Work out the finished part from the listing and answer in its coordinate system (mm). Face numbers are marked on the shaded views. A direction names the side the tool comes from. Give positions to 0.01 mm unless a question says otherwise; leave off trailing zeros. Order: outer loops, then holes, each group sorted by start corner. A loop starts at its lowest first (then second) coordinate and runs counter-clockwise, first axis right, second up. Notation, with made-up numbers: M 25.5,72.25 L 38.5,72.25 A29 cw 38.5,95.25 Z; hole C 72,48.5 d1. An arc over 180 degrees is marked long. One line per item, written item: value.
Autodesk Fusion 360 part; units mm, degrees
sketch "Sketch1" plane through (0, 0, 0) normal (0, 0, 1) x (1, 0, 0)
  line L0 (0, 0) -> (101.6, 0)
  line L1 (101.6, 0) -> (101.6, -76.2)
  line L2 (101.6, -76.2) -> (0, -76.2)
  line L3 (0, -76.2) -> (0, 0)
  line L4 (101.6, 0) -> (126.0466, 6.8938)
  line L5 (126.0466, 6.8938) -> (176.8466, 6.8938)
  line L6 (176.8466, 6.8938) -> (201.2932, 0)
  line L7 (201.2932, 0) -> (201.2932, -76.2)
  line L8 (201.2932, -76.2) -> (176.8466, -82.9718)
  line L9 (176.8466, -82.9718) -> (126.0466, -82.9718)
  line L10 (126.0466, -82.9718) -> (101.6, -76.2)
  dimension "d1" = 101.6
  dimension "d2" = 76.2
  dimension "d3" = 25.4
  dimension "d4" = 50.8
  dimension "d5" = 25.4
extrude "Extrude1" add sketch "Sketch1" along normal blind 12.7
fillet "Fillet1" radius 11.43 2 edges at (201.2932, -76.2, 6.35) (201.2932, 0, 6.35)
sketch "Sketch2" plane through (0, 0, 12.7) normal (0, 0, 1) x (-1, 0, 0)
  arc A0 (-201.2932, 8.6526) -> (-192.9654, -2.3484) centre (-189.8632, 8.6526) ccw
  line L0 (-192.9654, -2.3484) -> (-176.8466, -6.8938)
  line L1 (-176.8466, -6.8938) -> (-126.0466, -6.8938)
  line L2 (-126.0466, -6.8938) -> (-101.6, 0)
  line L3 (-101.6, 0) -> (0, 0)
  line L4 (0, 0) -> (0, 76.2)
  line L5 (0, 76.2) -> (-101.6, 76.2)
  line L6 (-101.6, 76.2) -> (-126.0466, 82.9718)
  line L7 (-126.0466, 82.9718) -> (-176.8466, 82.9718)
  line L8 (-176.8466, 82.9718) -> (-192.9144, 78.5209)
  arc A1 (-192.9144, 78.5209) -> (-201.2932, 67.5057) centre (-189.8632, 67.5057) ccw
  line L9 (-201.2932, 67.5057) -> (-201.2932, 8.6526)
  line L10 (0, 0) -> (-25.4, 0)
  line L11 (-25.4, 0) -> (-25.4, 6.35)
  line L12 (-25.4, 6.35) -> (0, 6.35)
  line L13 (0, 6.35) -> (0, 0)
  line L14 (0, 38.1) -> (-145.8184, 38.1) construction
  line L15 (-50.8, 0) -> (-50.8, 76.2) construction
  line L16 (0, 76.2) -> (-25.4, 76.2)
  line L17 (0, 69.85) -> (0, 76.2)
  line L18 (-25.4, 69.85) -> (0, 69.85)
  line L19 (-25.4, 76.2) -> (-25.4, 69.85)
  line L20 (-76.2, 0) -> (-76.2, 6.35)
  line L21 (-101.6, 0) -> (-76.2, 0)
  line L22 (-101.6, 6.35) -> (-101.6, 0)
  line L23 (-76.2, 6.35) -> (-101.6, 6.35)
  line L24 (-76.2, 69.85) -> (-101.6, 69.85)
  line L25 (-101.6, 69.85) -> (-101.6, 76.2)
  line L26 (-101.6, 76.2) -> (-76.2, 76.2)
  line L27 (-76.2, 76.2) -> (-76.2, 69.85)
  dimension "d10" = 25.4
  dimension "d11" = 6.35
extrude "Extrude2" add sketch "Sketch2" along normal blind 7.62 contours L3 L20 L21 L22 L23 | L5 L24 L25 L26 L27 | L3 L4 L10 L11 L12 L13 | L4 L5 L16 L17 L18 L19
sketch "Sketch3" plane through (0, -76.2, 0) normal (0, -1, 0) x (1, 0, 0)
  line L0 (0, 0) -> (101.6, 0)
  line L1 (101.6, 0) -> (101.6, 12.7)
  line L2 (101.6, 12.7) -> (101.6, 20.32)
  line L3 (101.6, 20.32) -> (76.2, 20.32)
  line L4 (76.2, 20.32) -> (76.2, 12.7)
  line L5 (76.2, 12.7) -> (25.4, 12.7)
  line L6 (25.4, 12.7) -> (25.4, 20.32)
  line L7 (25.4, 20.32) -> (0, 20.32)
  line L8 (0, 20.32) -> (0, 0)
  line L9 (2.54, 17.78) -> (22.86, 17.78)
  line L10 (22.86, 17.78) -> (22.86, 15.24)
  line L11 (22.86, 15.24) -> (2.54, 15.24)
  line L12 (2.54, 15.24) -> (2.54, 17.78)
  line L13 (78.74, 17.78) -> (99.06, 17.78)
  line L14 (99.06, 17.78) -> (99.06, 15.24)
  line L15 (99.06, 15.24) -> (78.74, 15.24)
  line L16 (78.74, 15.24) -> (78.74, 17.78)
extrude "Extrude3" cut sketch "Sketch3" against normal blind 86.36 contours L9 L10 L11 L12 | L13 L14 L15 L16
fillet "Fillet2" radius 3.81 8 edges at (101.6, -3.175, 20.32) (76.2, -3.175, 20.32) (101.6, -73.025, 20.32) (76.2, -73.025, 20.32) (25.4, -73.025, 20.32) (0, -73.025, 20.32) (0, -3.175, 20.32) (25.4, -3.175, 20.32)
sketch "Sketch4" plane through (0, 0, 12.7) normal (0, 0, 1) x (-1, 0, 0)
  line L0 (-101.6, 0) -> (-101.6, 6.35)
  line L1 (-101.6, 6.35) -> (-76.2, 6.35)
  line L2 (-76.2, 6.35) -> (-76.2, 0)
  line L3 (-76.2, 0) -> (-25.4, 0)
  line L4 (-25.4, 0) -> (-25.4, 6.35)
  line L5 (-25.4, 6.35) -> (0, 6.35)
  line L6 (0, 6.35) -> (0, 69.85)
  line L7 (0, 69.85) -> (-25.4, 69.85)
  line L8 (-25.4, 69.85) -> (-25.4, 76.2)
  line L9 (-25.4, 76.2) -> (-76.2, 76.2)
  line L10 (-76.2, 76.2) -> (-76.2, 69.85)
  line L11 (-76.2, 69.85) -> (-101.6, 69.85)
  line L12 (-101.6, 69.85) -> (-101.6, 76.2)
  line L13 (-101.6, 76.2) -> (-126.0466, 82.9718)
  line L14 (-126.0466, 82.9718) -> (-176.8466, 82.9718)
  line L15 (-176.8466, 82.9718) -> (-192.9144, 78.5209)
  arc A0 (-192.9144, 78.5209) -> (-201.2932, 67.5057) centre (-189.8632, 67.5057) ccw
  line L16 (-201.2932, 67.5057) -> (-201.2932, 8.6526)
  arc A1 (-201.2932, 8.6526) -> (-192.9654, -2.3484) centre (-189.8632, 8.6526) ccw
  line L17 (-192.9654, -2.3484) -> (-176.8466, -6.8938)
  line L18 (-176.8466, -6.8938) -> (-126.0466, -6.8938)
  line L19 (-126.0466, -6.8938) -> (-101.6, 0)
  circle A2 centre (-160.0534, 38.3696) radius 22.86
  dimension "d18" = 45.72
extrude "Extrude4" cut sketch "Sketch4" against normal blind 38.1 contours A2
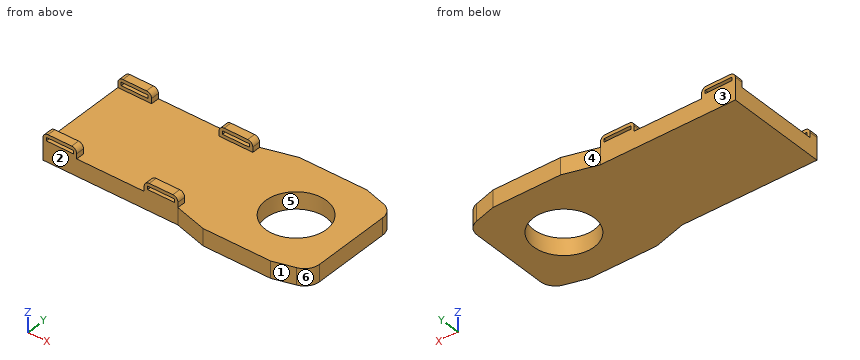
(1) Determine the mould class of the marked faces 3, 4, 5 and 6 for opening direction X: pulls with the +X half, pulls with the -X half, needs draft (parallel to the pull), parting line crosses it, or undercut.
Findings:
face 3: needs draft
face 4: pulls with the -X half
face 5: undercut
face 6: pulls with the +X half
(2) Section A-A, the plane x = 94 is taken. Give the vertices of the cut face in (y, z), then the cut area to 3 significant figures.
Findings:
outline: M -76.2,0 L 0,0 L 0,15.24 L -6.35,15.24 L -6.35,12.7 L -69.85,12.7 L -69.85,15.24 L -76.2,15.24 Z; M -76.2,17.78 L -69.85,17.78 L -69.85,20.32 L -76.2,20.32 Z; M -6.35,17.78 L 0,17.78 L 0,20.32 L -6.35,20.32 Z
area: 1,030 mm^2
(3) Section B-B, the plane y = -33.5 is taken. Give the vertices of the cut face in (x, z).
Findings:
outline: M 0,0 L 137.72,0 L 137.72,12.7 L 0,12.7 Z; M 182.39,0 L 201.29,0 L 201.29,12.7 L 182.39,12.7 Z
(4) Section C-C, the plane z = 6.25 is taken. Give the vertices of the cut face in (x, y), then the cut area to 3 significant figures.
Findings:
outline: M 0,-76.2 L 101.6,-76.2 L 126.05,-82.97 L 176.85,-82.97 L 192.91,-78.52 A11.43 ccw 201.29,-67.51 L 201.29,-8.65 A11.43 ccw 192.97,2.35 L 176.85,6.89 L 126.05,6.89 L 101.6,0 L 0,0 Z; hole C 160.05,-38.37 d45.72
area: 14,700 mm^2
(5) Find the intervals of material crossed by probe 1 along Y at (x, z) = (77, 17.5); probe 2 along Z at (x, y) = (84.5, -20); probe 3 along X at (y, z) = (-34, 3), in increasing order. Write a range as from..to.
Findings:
probe 1: y = -76.2..-69.85, -6.35..0
probe 2: z = 0..12.7
probe 3: x = 0..137.61, 182.49..201.29
(6) Which of the six approach directions +Z, -Z, +X, -X, +Y, -Y give full straight-line access (tool end or side, diameter ignored) to the marked faces 1 and 2?
Findings:
face 1: +Z, -Z, +X, -Y
face 2: +Z, -Z, -X, -Y
(7) Section D-D, the plane x = 146 is taken. Give the vertices of the cut face in (y, z), then the cut area to 3 significant figures.
Findings:
outline: M -82.97,0 L -56.4,0 L -56.4,12.7 L -82.97,12.7 Z; M -20.34,0 L 6.89,0 L 6.89,12.7 L -20.34,12.7 Z
area: 683 mm^2
(8) Given P1, Ø0.8, axis at y = -4.5, z = 17, coming from the -X side; P2, Ø3, axis at y = -73.5, z = 14.5, coming from the +X side; P3, Ø2.5, axis at x = 17.5, z = 15, coming from the +Y side; P4, Ø3, axis at x = 107.5, z = 7.5, coming from the -Y side, each flat-ended and moving along its own axis, determine where each tip first touches the part or whether it passes through.
Findings:
P1: stops at x = 0
P2: stops at x = 101.6
P3: stops at y = 0
P4: stops at y = -78.25
